from build123d import *

# Parameters (mm, degrees)
RIBCUT_START     = -0.2561
RIBCUT_DEPTH     = 0.2561
RIBCUTSPAT_COUNT = 8
RIBCUTSPAT_ANGLE = 315


with BuildPart() as part:
    # BodySke → BaseBody (revolve)
    with BuildSketch(Plane.XY, mode=Mode.PRIVATE) as basebody_sk:
        with BuildLine():
            Line((-0.64, 2.944), (-0.64, 0))
            Line((-0.64, 0), (18, 0))
            Line((18, 0), (18, 2.055))
            Line((18, 2.055), (17.555, 2.5))
            Line((17.555, 2.5), (0.25854, 2.5))
            Line((0.25854, 2.5), (0.25854, 2.94146))
            ThreePointArc((0.25854, 2.94146), (0.183559336, 3.122479336), (0.00254, 3.19746))
            Line((0.00254, 3.19746), (0, 3.19746))
            Line((0, 3.19746), (0, 3.2))
            Line((0, 3.2), (-0.384, 3.2))
            ThreePointArc((-0.384, 3.2), (-0.565019336, 3.125019336), (-0.64, 2.944))
        make_face()
    revolve(basebody_sk.sketch.rotate(Axis((0, 0, 0), (1, 0, 0)), 90), axis=Axis((0, 0, 0), (1, 0, 0)))

    # RibCutSke → RibCut (cut)
    with BuildSketch(Plane(origin=(0.25854, 1.794401132, -0.090952894), x_dir=(0, 0, -1), z_dir=(1, 0, 0)).offset(RIBCUT_START)):
        with BuildLine():
            Line((0.300133268, 1.028638296), (0.300133268, 1.381610771))
            ThreePointArc((0.300133268, 1.381610771), (1.133634089, 1.162013372), (1.878286983, 0.7279181))
            Line((1.878286983, 0.7279181), (1.628697752, 0.478328869))
            ThreePointArc((1.628697752, 0.478328869), (0.999694888, 0.838655535), (0.300133268, 1.028638296))
        make_face()
    ribcut = extrude(amount=RIBCUT_DEPTH, mode=Mode.SUBTRACT)

    # RibCutsPat: RibCut ×8 about axis
    ribcutspat_axis = Axis((0, 0, 0), (1, 0, 0))
    for i in range(1, RIBCUTSPAT_COUNT):
        add(ribcut.rotate(ribcutspat_axis, i * RIBCUTSPAT_ANGLE / (RIBCUTSPAT_COUNT - 1)), mode=Mode.SUBTRACT)


solid = part.part
Here's how the part is built. I have some questions about the finished solid (model axes, mm). A direction names the side the tool comes from. Round coordinates to 2 decimals unless told otherwise and drop trailing zeros. Order: outer loops, then holes, each group sorted by start corner. A loop starts at its lowest first (then second) coordinate and runs counter-clockwise, first axis right, second up. Notation, with made-up numbers: (56.25, 16.25) -> (94.25, 16.25) arc R23 cw to (94.25, 28.25) -> close; hole circle Ø5 at (-33.75, -39.5). An arc over 180 degrees is marked (long way). Use CSV: the item, a comma, the result in double quotes.
1. Which directions (+Z, -Z, +X, -X, +Y, -Y) give clear straight access to the entire face, cutting with the end or side of a thin tool? Please do faces 1 (the face through (-0.195, -0.961, 3.052)), 2 (the face through (0.002, 1.1, -2.8)), 3 (the face through (0.002, -1.1, 2.8)).
Recorded:
face 1,"+X, -X"
face 2,"-Z, +X"
face 3,"+Z, +X"
2. I want a section at C-C on x = 10. List the corners of the cut face in (y, z) for me.
Recorded:
outline,"circle Ø5 at (0, 0)"
3. I need wall thicknesses on line 1 along Z through (x, y) = (8.25, -1.75); line 2 along Y through (x, z) = (13.5, 0). Which ranges of each line are inside material? Lowest first, please.
Recorded:
line 1,"z = -1.79 to 1.79"
line 2,"y = -2.5 to 2.5"
4. I'm going to push flat-ended pins straight in: P1, Ø1, axis at x = 16, z = -2, coming from the -Y side; P2, Ø1, axis at x = 4.5, y = 2, coming from the -Z side; P3, Ø3, axis at x = 4.5, y = 1.5, coming from the -Z side. Where does each tip first touch, or does it pass through?
Recorded:
P1,"stops at y = -2"
P2,"stops at z = -2"
P3,"stops at z = -2.5"
5. Thinking about a two-plate mould opening in Z: for faces 4 (the face through (0.002, -2.8, -1.1)), 5 (the face through (0.002, 2.8, 1.1)), 6 (the face through (18, 0, 0)), 7 (the face through (8.8, -0.1, -2.5)), which applies, pulls with the +Z half, pulls with the -Z half, needs draft (parallel to the pull), parting line crosses it, or undercut?
Recorded:
face 4,"undercut"
face 5,"undercut"
face 6,"needs draft"
face 7,"parting line crosses it"
